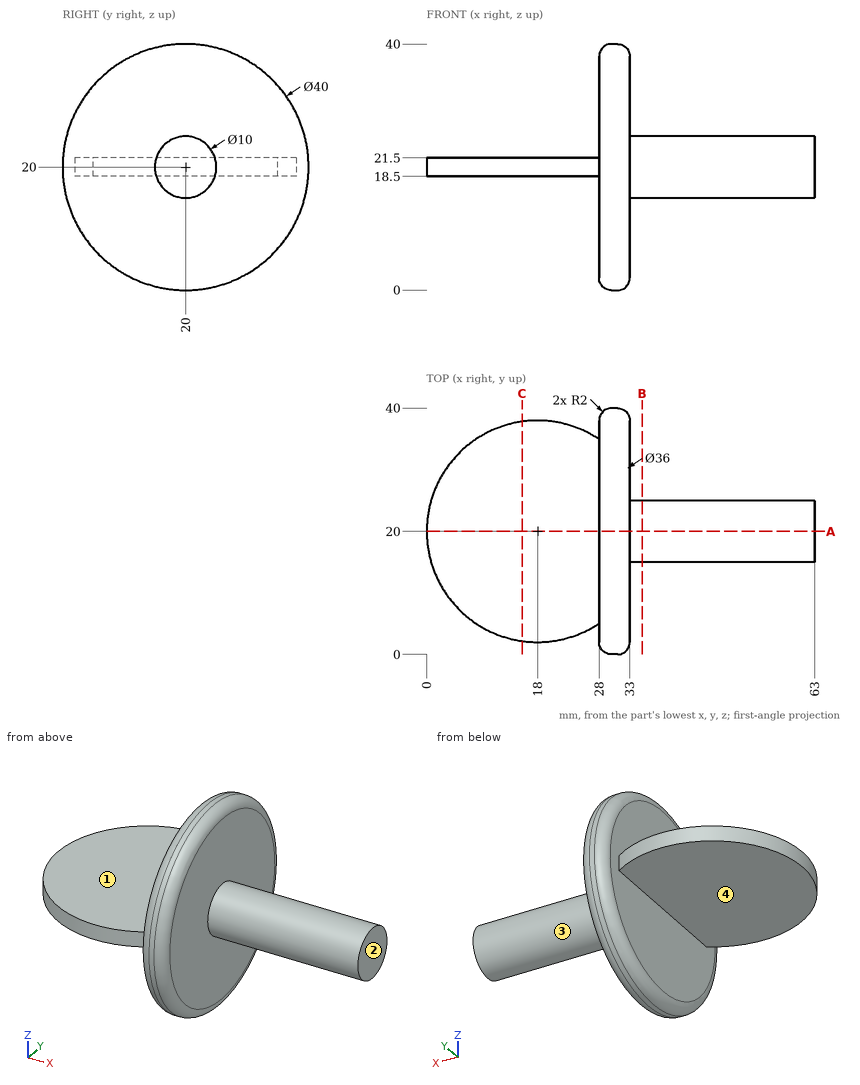
For this review, use the dimensioned drawing (mm, ordinates from the lowest corner) and the shaded views. A direction names the side the tool comes from. Give positions to 0.01 mm unless a question says otherwise; leave off trailing zeros. Loops run counter-clockwise (first coordinate to the right, second up) from the corner with the lowest first, then second, coordinate; pieces in that order, holes last.
Item 1: Insertion check: pin 1 (12 mm diameter, centred on y = 6.5, z = 33.5, fed in from -X); pin 2 (2 mm diameter, centred on y = 17.5, z = 32, fed in from +X); pin 3 (1.5 mm diameter, centred on y = 19, z = 19.5, fed in from -X). Each pin has a flat end and moves straight along its axis. Give the tip position at first contact, or say it passes through.
Item 2: Take a section at B-B, the plane x = 35. State the section outline as (y, z) points, and give its area (3 significant figures).
Item 3: Take a section at A-A, the plane y = 20. State the section outline as (x, z) points, and give its area (3 significant figures).
Item 4: For line 1 along X through (y, z) = (25, 28); line 2 along Z through (x, y) = (27, 9); line 3 along X through (y, z) = (20, 22), list the stretches that pass through material, from the lowest coordinate up.
Item 5: Take a section at C-C, the plane x = 15.5. State the section outline as (y, z) points, and give its area (3 significant figures).
Item 6: Tool access review of the marked faces 1, 2, 3 and 4: name each direction out of +Z, -Z, +X, -X, +Y, -Y from which nothing blocks a thin tool from reaching the whole face with its end or side.
Calculated:
1. pin 1: stops at x = 28
1. pin 2: stops at x = 33
1. pin 3: stops at x = 0
2. outline: circle Ø10 at (20, 20)
2. area: 78.5 mm2
3. outline: (0, 18.5) - (28, 18.5) - (28, 2) arc R2 ccw to (30, 0) - (31, 0) arc R2 ccw to (33, 2) - (33, 15) - (63, 15) - (63, 25) - (33, 25) - (33, 38) arc R2 ccw to (31, 40) - (30, 40) arc R2 ccw to (28, 38) - (28, 21.5) - (0, 21.5) - close
3. area: 581 mm2
4. line 1: x = 28 to 33
4. line 2: z = 18.5 to 21.5
4. line 3: x = 28 to 63
5. outline: (2.17, 18.5) - (37.83, 18.5) - (37.83, 21.5) - (2.17, 21.5) - close
5. area: 107 mm2
6. face 1: +Z, -X, +Y, -Y
6. face 2: +Z, -Z, +X, +Y, -Y
6. face 3: +X
6. face 4: -Z, -X, +Y, -Y
